Build history of the part. All positions in model axes, mm. Face numbers are marked on the shaded views. A direction names the side the tool comes from. Give positions to 0.01 mm unless a question says otherwise; leave off trailing zeros. Write each loop counter-clockwise with the first axis right and the second up, starting at its lowest first coordinate (ties: lowest second). Pieces come first, ordered by that corner, then holes. Notation, with made-up numbers: M 15,27 L 32,27 A18 cw 32,55 Z; hole C 53,8 d1. An arc over 180 degrees is marked long. Return JSON: item names as keys, results as strings. Group by question number.
Q1. Flat gauge pins, fed straight in: pin 1 Ø1 at (y, z) = (124, 46) entering from -X; pin 2 Ø1 at (x, z) = (-1202.5, 61.5) entering from +Y. Where does each tip first touch, or does it go through?
Q2. Tool access for the marked faces 1, 2 and 3: list every direction of +Z, -Z, +X, -X, +Y, -Y with a clear straight run to the whole face (end or side of a thin tool).
Q3. Wall check: probe 1 along Y at (x, z) = (-164, 60); probe 2 along Y at (x, z) = (-934.5, 20); probe 3 along X at (y, z) = (166, 26.5). Give the ranges that are in metal, low to high.
Q4. Band-saw the part on A-A, the plane z = 48.5. Give the cut face in (x, y).
Q5. Band-saw the part on C-C, the plane y = 219. Give the cut face in (x, z), then the cut area to 3 significant figures.
Q6. Band-saw the part on B-B, the plane x = -316. Give the cut face in (y, z), then the cut area to 3 significant figures.
from build123d import *

# Parameters (mm, degrees)
F1_DEPTH = 76.2


with BuildPart() as f1:
    # F0 (on Top) → F1 (new body)
    with BuildSketch(Plane.XY):
        with BuildLine():
            Line((-799.919396, 0), (0, 0))
            Line((0, 0), (0, 342.9))
            Line((0, 342.9), (-466.619206, 342.9))
            Line((-466.619206, 342.9), (-774.7, 425.45))
            Line((-774.7, 425.45), (-1151.629547, 425.45))
            Line((-1151.629547, 425.45), (-1333.5, 320.447045))
            ThreePointArc((-1333.5, 320.447045), (-1346.2, 298.45), (-1333.5, 276.452955))
            Line((-1333.5, 276.452955), (-1151.629547, 171.45))
            Line((-1151.629547, 171.45), (-915.677907, 171.45))
            ThreePointArc((-915.677907, 171.45), (-893.824645, 164.559693), (-879.875618, 146.380967))
            Line((-879.875618, 146.380967), (-835.721685, 25.069033))
            ThreePointArc((-835.721685, 25.069033), (-821.772658, 6.890307), (-799.919396, 0))
        make_face()
    extrude(amount=F1_DEPTH)


solid = f1.part
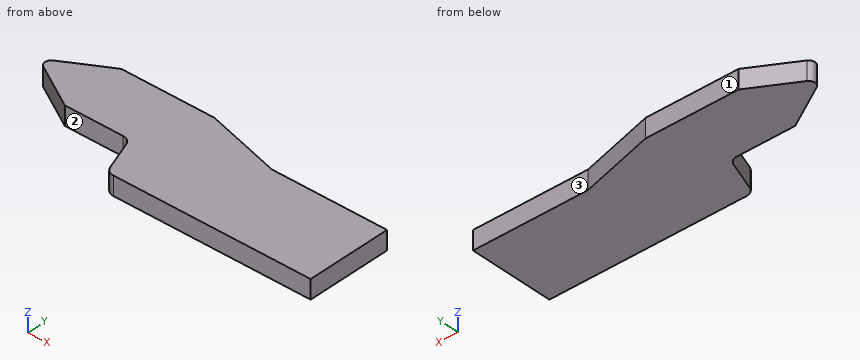
From the geometry:
{
 "1": {"pin 1": "stops at x = -871.91", "pin 2": "stops at y = 396.37"},
 "2": {"face 1": "+Z, -Z, +X, -X, +Y", "face 2": "+Z, -Z, -X, -Y", "face 3": "+Z, -Z, +X, +Y"},
 "3": {"probe 1": "y = 0 to 342.9", "probe 2": "y = 171.45 to 425.45", "probe 3": "x = -896.04 to 0"},
 "4": {"outline": "M -1333.5,276.45 L -1151.63,171.45 L -915.68,171.45 A38.1 cw -879.88,146.38 L -835.72,25.07 A38.1 ccw -799.92,0 L 0,0 L 0,342.9 L -466.62,342.9 L -774.7,425.45 L -1151.63,425.45 L -1333.5,320.45 A25.4 ccw Z"},
 "5": {"outline": "M -1233.99,0 L 0,0 L 0,76.2 L -1233.99,76.2 Z", "area": "94,000 mm^2"},
 "6": {"outline": "M 0,0 L 342.9,0 L 342.9,76.2 L 0,76.2 Z", "area": "26,100 mm^2"}
}
